```python
from build123d import *

# Parameters (mm, degrees)
SKETCH1_W           = 40
SKETCH1_H           = 20
BOSS_EXTRUDE1_DEPTH = 26.5
SKETCH2_W           = 52.8
SKETCH2_H           = 20
BOSS_EXTRUDE2_DEPTH = 2.5
SKETCH3_W           = 40
SKETCH3_H           = 20
BOSS_EXTRUDE3_DEPTH = 7.3
SKETCH4_R           = 6.5
BOSS_EXTRUDE4_DEPTH = 1.3


with BuildPart() as part:
    # Sketch1 → Boss-Extrude1 (new body)
    with BuildSketch(Plane(origin=(0, 0, 0), x_dir=(1, 0, 0), z_dir=(0, 1, 0))):
        Rectangle(SKETCH1_W, SKETCH1_H)
    extrude(amount=BOSS_EXTRUDE1_DEPTH)

    # Sketch2 → Boss-Extrude2 (add)
    with BuildSketch(Plane(origin=(0, 26.5, 0), x_dir=(1, 0, 0), z_dir=(0, 1, 0))):
        Rectangle(SKETCH2_W, SKETCH2_H)
    extrude(amount=BOSS_EXTRUDE2_DEPTH)

    # Sketch3 → Boss-Extrude3 (add)
    with BuildSketch(Plane(origin=(0, 29, 0), x_dir=(1, 0, 0), z_dir=(0, 1, 0))):
        Rectangle(SKETCH3_W, SKETCH3_H)
    extrude(amount=BOSS_EXTRUDE3_DEPTH)

    # Sketch4 → Boss-Extrude4 (add)
    with BuildSketch(Plane(origin=(0, 36.3, 0), x_dir=(1, 0, 0), z_dir=(0, 1, 0))):
        with Locations((-10.5, 0)):
            Circle(SKETCH4_R)
    extrude(amount=BOSS_EXTRUDE4_DEPTH)


solid = part.part
```
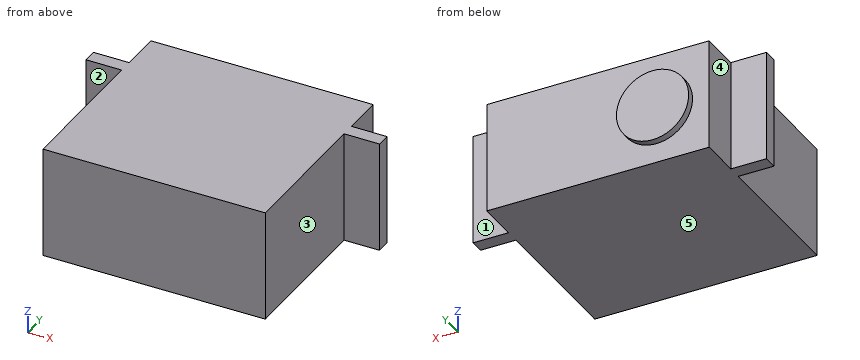
Can you work these out from the model? Positions are in its coordinate system, mm. Face numbers are marked on the shaded views. A direction names the side the tool comes from. Coordinates: 2 decimals unless noted, no trailing zeros. Order: outer loops, then holes, each group sorted by start corner. A loop starts at its lowest first (then second) coordinate and runs counter-clockwise, first axis right, second up.
1. I need wall thicknesses on line 1 (Y direction, x = 16, z = 8); line 2 (X direction, y = 22.5, z = 6.75); line 3 (Y direction, x = -21.5, z = -9). Which ranges of each line are inside material? Lowest first, please.
2. I'm going to push flat-ended pins straight in: pin 1 (4 mm diameter, centred on y = 32, z = -7.5, fed in from -X); pin 2 (4 mm diameter, centred on x = 12, z = 4, fed in from +Y); pin 3 (6 mm diameter, centred on y = 33.5, z = 2, fed in from +X). Where does each tip first touch, or does it pass through?
3. If we section it at B-B (x = -22): Please give me the cut outline in (y, z).
4. If we section it at A-A (z = 0): Please give me the cut outline in (x, y), then the cut area to 3 significant figures.
5. If we section it at C-C (y = 13): Please give me the cut outline in (x, z), then the cut area to 3 significant figures.
6. If we section it at D-D (z = 2.75): Please give me the cut outline in (x, y), then the cut area to 3 significant figures.
7. For the marked faces 1, 2, 3, 4 and 5, which set-ups out of +Z, -Z, +X, -X, +Y, -Y let a thin tool reach every point of the face, with its end or its side?
Entries:
1. line 1: y = 0 to 36.3
1. line 2: x = -20 to 20
1. line 3: y = 26.5 to 29
2. pin 1: stops at x = -20
2. pin 2: stops at y = 36.3
2. pin 3: stops at x = 20
3. outline: (26.5, -10) - (29, -10) - (29, 10) - (26.5, 10) - close
4. outline: (-26.4, 26.5) - (-20, 26.5) - (-20, 0) - (20, 0) - (20, 26.5) - (26.4, 26.5) - (26.4, 29) - (20, 29) - (20, 36.3) - (-4, 36.3) - (-4, 37.6) - (-17, 37.6) - (-17, 36.3) - (-20, 36.3) - (-20, 29) - (-26.4, 29) - close
4. area: 1,500 mm2
5. outline: (-20, -10) - (20, -10) - (20, 10) - (-20, 10) - close
5. area: 800 mm2
6. outline: (-26.4, 26.5) - (-20, 26.5) - (-20, 0) - (20, 0) - (20, 26.5) - (26.4, 26.5) - (26.4, 29) - (20, 29) - (20, 36.3) - (-4.61, 36.3) - (-4.61, 37.6) - (-16.39, 37.6) - (-16.39, 36.3) - (-20, 36.3) - (-20, 29) - (-26.4, 29) - close
6. area: 1,500 mm2
7. face 1: +Z, -Z, +X, +Y
7. face 2: +Z, -Z, -X, -Y
7. face 3: +Z, -Z, +X, -Y
7. face 4: +Z, -Z, -X, +Y
7. face 5: -Z, +X, -X, +Y, -Y
